Autodesk Inventor part; units mm, degrees
ref_plane "YZ Plane" through (0, 0, 0) normal (1, 0, 0) x (0, 1, 0)
ref_plane "XZ Plane" through (0, 0, 0) normal (0, 1, 0) x (-1, 0, 0)
ref_plane "XY Plane" through (0, 0, 0) normal (0, 0, 1) x (1, 0, 0)
sketch "Szkic1" plane through (0, 0, 0) normal (0, 0, 1) x (1, 0, 0)
  line L0 (-30, -19) -> (30, -19)
  line L1 (30, -19) -> (30, 19)
  line L2 (30, 19) -> (-30, 19)
  line L3 (-30, 19) -> (-30, -19)
  line L4 (-30, -19) -> (30, 19) construction
  line L5 (30, -19) -> (-30, 19) construction
  line L6 (0, 19) -> (0, 1)
  circle A0 centre (0, 1) radius 15
  point P0 (0, 0)
  dimension "d0" = 60
  dimension "d1" = 38
  dimension "d2" = 18
  dimension "d3" = 30
extrude "Wyciągnięcie proste1" add sketch "Szkic1" along normal blind 8
sketch "Szkic2" plane through (0, 0, 8) normal (0, 0, 1) x (1, 0, 0)
  circle A0 centre (0, 1) radius 15
  line L0 (-30, -19) -> (30, -19)
  line L1 (30, -19) -> (30, 19)
  line L2 (30, 19) -> (-30, 19)
  line L3 (-30, 19) -> (-30, -19)
  line L4 (-30, 19) -> (-30, -19)
  line L5 (-30, 19) -> (-22, 19)
  line L6 (30, 19) -> (-30, 19)
  line L7 (-22, 19) -> (-22, -19)
  line L8 (30, 19) -> (22, 19)
  line L9 (22, 19) -> (22, -19)
  line L10 (-22, 19) -> (-22, 11)
  line L11 (-22, -19) -> (-22, -11)
  line L12 (22, 19) -> (22, 11)
  line L13 (22, -19) -> (22, -11)
  circle A1 centre (-22, 11) radius 2.5
  circle A2 centre (-22, -11) radius 2.5
  circle A3 centre (22, 11) radius 2.5
  circle A4 centre (22, -11) radius 2.5
  point P0 (0, 0)
  dimension "d6" = 8
  dimension "d7" = 8
  dimension "d8" = 8
  dimension "d9" = 8
  dimension "d10" = 8
  dimension "d11" = 8
  dimension "d12" = 5
  dimension "d13" = 5
  dimension "d14" = 5
  dimension "d15" = 5
extrude "Wyciągnięcie proste2" cut sketch "Szkic2" against normal up to next contours A2 L7 | L7 A2 | A4 L9 | L9 A4 | A1 L7 | L7 A1 | A3 L9 | L9 A3
properties part number "Uchwyt silnika krokowego osi X - płaski (blacha łożyska)"
Here's how the part is built. I have some questions about the finished solid (model axes, mm). Round coordinates to 2 decimals unless told otherwise and drop trailing zeros. Order: outer loops, then holes, each group sorted by start corner. A loop starts at its lowest first (then second) coordinate and runs counter-clockwise, first axis right, second up. Notation, with made-up numbers: M -6.5,86.25 L 43.5,86.25 A28 ccw 43.5,123.25 Z; hole C -7,64.5 d11. An arc over 180 degrees is marked long. Return JSON: item names as keys, results as strings. Group by question number.
1. Please list where these lines run through material, in increasing order: probe 1 along Y at (x, z) = (22, 2.25); probe 2 along Y at (x, z) = (20.5, 2.25); probe 3 along X at (y, z) = (9.5, 7.5).
2. If we mould it in two halves opening along X, with no side actions, what happens to faces 1 (the face through (30, 0, 4)), 2 (the face through (0, 19, 4)), 3 (the face through (-24, 9.5, 4.1)), 4 (the face through (-30, 0, 4))? For each: pulls with the +X half, pulls with the -X half, needs draft (parallel to the pull), parting line crosses it, or undercut.
3. If we section it at B-B on x = 0: List the corners of the cut face in (y, z) for me.
4. If we section it at A-A on y = -11: List the corners of the cut face in (x, z) for me, then the cut area to 3 significant figures.
5. If we section it at C-C on x = 22: List the corners of the cut face in (y, z) for me, then the cut area to 3 significant figures.
6. I'm going to push a flat-ended pin straight in: pin 1 Ø4 at (x, y) = (-22, -11) entering from -Z. Where does the tip first touch, or does it pass through?
7. If we section it at D-D on z = 4.5: List the corners of the cut face in (x, y) for me.
Reply:
{
 "1": {"probe 1": "-19 to -13.5, -8.5 to 8.5, 13.5 to 19", "probe 2": "-19 to -13, -9 to 9, 13 to 19", "probe 3": "-30 to -24, -20 to -12.36, 12.36 to 20, 24 to 30"},
 "2": {"face 1": "pulls with the +X half", "face 2": "needs draft", "face 3": "undercut", "face 4": "pulls with the -X half"},
 "3": {"outline": "M -19,0 L -14,0 L -14,8 L -19,8 Z; M 16,0 L 19,0 L 19,8 L 16,8 Z"},
 "4": {"outline": "M -30,0 L -24.5,0 L -24.5,8 L -30,8 Z; M -19.5,0 L -9,0 L -9,8 L -19.5,8 Z; M 9,0 L 19.5,0 L 19.5,8 L 9,8 Z; M 24.5,0 L 30,0 L 30,8 L 24.5,8 Z", "area": "256 mm^2"},
 "5": {"outline": "M -19,0 L -13.5,0 L -13.5,8 L -19,8 Z; M -8.5,0 L 8.5,0 L 8.5,8 L -8.5,8 Z; M 13.5,0 L 19,0 L 19,8 L 13.5,8 Z", "area": "224 mm^2"},
 "6": {"pin 1": "through"},
 "7": {"outline": "M -30,-19 L 30,-19 L 30,19 L -30,19 Z; hole C -22,-11 d5; hole C -22,11 d5; hole C 0,1 d30; hole C 22,-11 d5; hole C 22,11 d5"}
}
